```python
from build123d import *

# Parameters (mm, degrees)
F0_W     = 101.6
F0_H     = 101.6
F1_DEPTH = 101.6
F2_R     = 25.4
F3_DEPTH = 101.6
F6_W     = 50.8
F6_H     = 50.8
F7_DEPTH = 101.6
F8_R     = 6.35


with BuildPart() as f1:
    # F0 (on Top) → F1 (new body)
    with BuildSketch(Plane.XY):
        with Locations((0.3681425005, 0.5443057779)):
            Rectangle(F0_W, F0_H)
    extrude(amount=F1_DEPTH)

    # F2 (on face) → F3 (join)
    with BuildSketch(Plane.XY.offset(101.6)):
        Circle(F2_R)
    extrude(amount=F3_DEPTH)

    # F4 (on face) → F5 (revolve)
    with BuildSketch(Plane.XY.offset(203.2)):
        with BuildLine():
            Line((25.4, 0), (38.1, 0))
            ThreePointArc((38.1, 0), (0, 38.1), (-38.1, 0))
            Line((-38.1, 0), (-25.4, 0))
            ThreePointArc((-25.4, 0), (0, 25.4), (25.4, 0))
        make_face()
    revolve(axis=Axis((0, 0, 203.2), (1, 0, 0)))

    # F6 (on face) → F7 (cut)
    with BuildSketch(Plane(origin=(0, 51.3443057779, 0), x_dir=(-1, 0, 0), z_dir=(0, 1, 0))):
        with Locations((0, 49.2945600852)):
            Rectangle(F6_W, F6_H)
    extrude(amount=-F7_DEPTH, mode=Mode.SUBTRACT)

    # F8
    f8_edges = [f1.edges().sort_by_distance(p)[0] for p in [
        (51.168143, 0.544306, 101.6),
        (0.368143, 51.344306, 101.6),
        (51.168143, -50.255694, 50.8),
        (51.168143, 51.344306, 50.8),
        (51.168143, 0.544306, 0),
        (0.368143, 51.344306, 0),
        (-50.431857, 51.344306, 50.8),
        (-25.4, 0, 174.801937),
        (-25.4, 0, 101.6),
        (0.368143, -50.255694, 101.6),
        (-50.431857, -50.255694, 50.8),
        (0.368143, -50.255694, 0),
        (-50.431857, 0.544306, 101.6),
        (-50.431857, 0.544306, 0),
    ]]
    fillet(f8_edges, radius=F8_R)


solid = f1.part
```
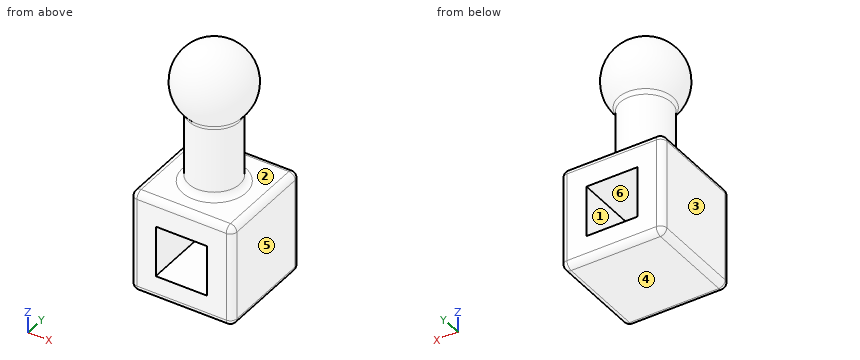
Can you work these out from the model? Positions are in its coordinate system, mm. Face numbers are marked on the shaded views. A direction names the side the tool comes from. Give positions to 0.01 mm unless a question says otherwise; leave off trailing zeros. Write each loop counter-clockwise with the first axis right and the second up, starting at its lowest first coordinate (ties: lowest second). Pieces come first, ordered by that corner, then holes. Notation, with made-up numbers: (-30, 42.5) -> (-18, 42.5) arc R20 ccw to (-18, 76.5) -> close; hole circle Ø4 at (55.25, 62.5). An arc over 180 degrees is marked (long way). One line per item, written item: value.
Q1. We'd pull the mould along Z, two halves only. Please class the marked faces 4, 5 and 6: +Z half, -Z half, draft (parallel to the pull), parting line (faces both ways), or undercut.
Results found:
face 4: -Z half
face 5: draft
face 6: undercut
Q2. Imagine slicing it at A-A on x = 0. Give the number of separate pieces and of enclosed holes in the cut face, and give its area (3 significant figures).
Results found:
separate pieces: 2
enclosed holes: 1
area: 12,100 mm^2
Q3. Please list where these lines run through material, in increasing order: line 1 (X direction, y = 26, z = 59); line 2 (Z direction, x = 9.5, y = -21); line 3 (Z direction, x = -18, y = 26). Write a range as [from, to].
Results found:
line 1: x = [-50.43, -25.4], [25.4, 51.17]
line 2: z = [0, 23.89], [74.69, 203.2], [213.87, 233.54]
line 3: z = [0, 23.89], [74.69, 101.6], [181.95, 224.45]
Q4. Which directions (+Z, -Z, +X, -X, +Y, -Y) give clear straight access to the entire face, cutting with the end or side of a thin tool? Please do the marked faces 1, 2 and 3.
Results found:
face 1: +Y, -Y
face 2: none
face 3: +Z, -Z, -X, +Y, -Y
Q5. Imagine slicing it at C-C on x = 41. Please give me the cut outline in (y, z), and give its area (3 significant figures).
Results found:
outline: (-50.26, 6.35) arc R6.35 ccw to (-43.91, 0) -> (44.99, 0) arc R6.35 ccw to (51.34, 6.35) -> (51.34, 95.25) arc R6.35 ccw to (44.99, 101.6) -> (-43.91, 101.6) arc R6.35 ccw to (-50.26, 95.25) -> close
area: 10,300 mm^2
Q6. Imagine slicing it at D-D on z = 158. Please give me the cut outline in (x, y), and give its area (3 significant figures).
Results found:
outline: circle Ø50.8 at (0, 0)
area: 2,030 mm^2
Q7. For P1, Ø8, axis at y = -3, z = 118.5, coming from the -X side; P2, Ø5, axis at y = -12.5, z = 132.5, coming from the -X side; P3, Ø5, axis at y = 11.5, z = 204, coming from the +X side (3 decimals), each with a flat end and sliding along its axis, tell me the tip position at first contact or that it passes through.
Results found:
P1: stops at x = -25.4
P2: stops at x = -23.35
P3: stops at x = 37.015
